For this review, take the finished solid that the model builds, in its own axes (mm). Face numbers are marked on the shaded views. Round coordinates to 2 decimals unless told otherwise and drop trailing zeros. Order: outer loops, then holes, each group sorted by start corner. A loop starts at its lowest first (then second) coordinate and runs counter-clockwise, first axis right, second up. Notation, with made-up numbers: (42.5, 67.25) -> (91.5, 67.25) arc R18 ccw to (91.5, 72.25) -> close; hole circle Ø7 at (8.5, -30). An arc over 180 degrees is marked (long way). Use a Markdown table: item, result. Add a question column.
1) Consider section B-B (y = 0). State the section outline as (x, z) points, plus the area to 4 significant figures.
2) Wall thickness on line 1 along Z through (x, y) = (2.25, 2.5); line 2 along X through (y, z) = (4, 3.2); line 3 along Y through (x, z) = (-4, 3.85): over which ranges is each line inside the solid? List them lowest first. Write a range as [from, to].
3) Draft analysis for pull direction X (two halves, no side actions). For the marked faces 1, 2 and 3, state which applies: pulls with the +X half, pulls with the -X half, needs draft (parallel to the pull), parting line crosses it, or undercut.
4) Clearance check with a flat-ended pin moving along its axis: P1, Ø1, axis at x = 2, y = 0.5, coming from the +Z side. State where the tip first meets the part, or that it passes through.
5) Consider section A-A (x = 0). State the section outline as (y, z) points.
6) Consider section C-C (x = 4.75). State the section outline as (y, z) points.
```python
from build123d import *

# Parameters (mm, degrees)
EXTRUDE_1_DEPTH     = 4
FILLET_1_R          = 1.5
SKETCH_2_R          = 4.25
CUT_EXTRUDE_1_DEPTH = 0.1


with BuildPart() as part:
    # Эскиз1 → Бобышка-Вытянуть1 (new body)
    with BuildSketch(Plane.XY):
        Polygon((-5, 4.545941546), (-5, -5.1), (4.445941546, -5.1), (5, -4.545941546), (5, 5.1), (-4.445941546, 5.1), align=None)
    extrude(amount=EXTRUDE_1_DEPTH)

    # Скругление1
    fillet_1_edges = [part.edges().sort_by_distance(p)[0] for p in [
        (5, 5.1, 2),
        (-5, -5.1, 2),
    ]]
    fillet(fillet_1_edges, radius=FILLET_1_R)

    # Эскиз2 → Вырез-Вытянуть1 (cut)
    with BuildSketch(Plane.XY.offset(4)):
        Circle(SKETCH_2_R)
    extrude(amount=-CUT_EXTRUDE_1_DEPTH, mode=Mode.SUBTRACT)


solid = part.part
```
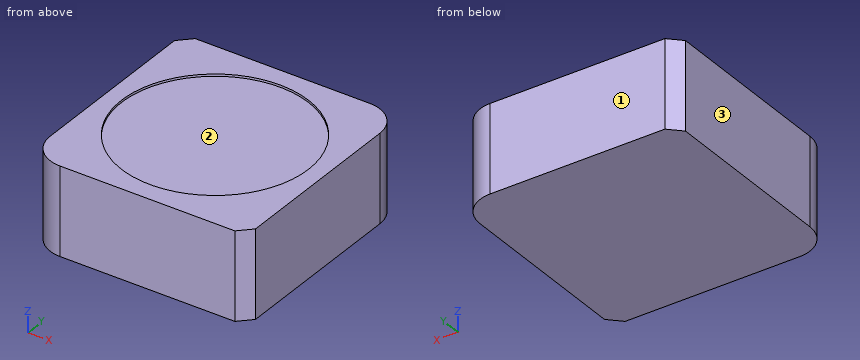
Results list:
| question | item | result |
|---|---|---|
| 1 | outline | (-5, 0) -> (5, 0) -> (5, 4) -> (4.25, 4) -> (4.25, 3.9) -> (-4.25, 3.9) -> (-4.25, 4) -> (-5, 4) -> close |
| 1 | area | 39.15 mm2 |
| 2 | line 1 | [0, 3.9] |
| 2 | line 2 | [-5, 4.95] |
| 2 | line 3 | [-5.01, 5.1] |
| 3 | face 1 | needs draft |
| 3 | face 2 | undercut |
| 3 | face 3 | pulls with the -X half |
| 4 | P1 | z = 3.9 |
| 5 | outline | (-5.1, 0) -> (5.1, 0) -> (5.1, 4) -> (4.25, 4) -> (4.25, 3.9) -> (-4.25, 3.9) -> (-4.25, 4) -> (-5.1, 4) -> close |
| 6 | outline | (-4.8, 0) -> (4.43, 0) -> (4.43, 4) -> (-4.8, 4) -> close |
